Check sheet for the drawn part. Datum: minimum x, y, z corner. Units: mm. A direction names the side the tool comes from. Give positions to 0.01 mm unless a question says otherwise; leave off trailing zeros. Order: outer loops, then holes, each group sorted by start corner. A loop starts at its lowest first (then second) coordinate and runs counter-clockwise, first axis right, second up. Notation, with made-up numbers: (22.5, 81.5) -> (64.5, 81.5) arc R19 cw to (64.5, 92.5) -> close; hole circle Ø9 at (25.5, -33). An arc over 180 degrees is marked (long way). One line per question, with ' | ' between items. Start each with the question number.
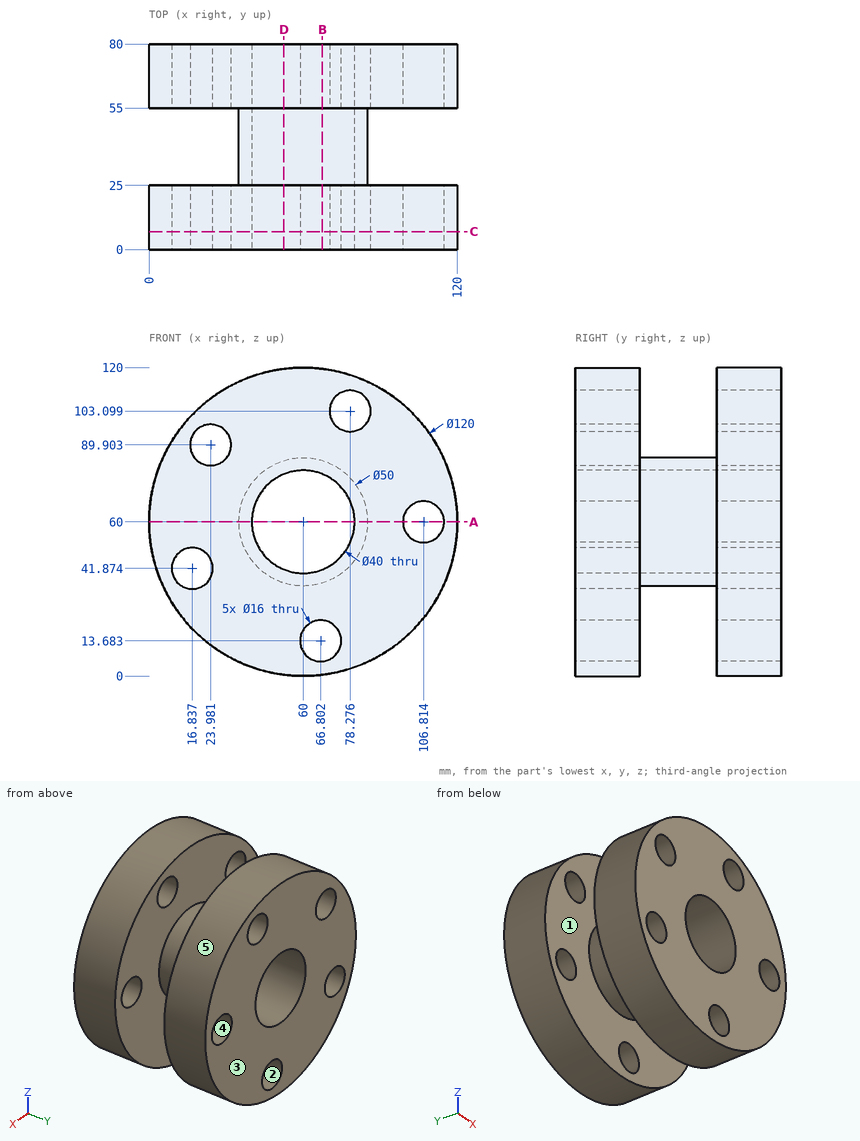
1. Cross-section at D-D on x = 52.5. Record the boundary of the cut face in (y, z).
2. Scan lines: probe 1 along Y at (x, z) = (79.5, 20); probe 2 along X at (y, z) = (68.5, 64.5) (1 decimal); probe 3 along Z at (x, y) = (20, 19.5) (1 decimal). Record each from-to range of solid material in increasing order.
3. Cross-section at C-C on y = 7. Record the boundary of the cut face in (x, z) (1 decimal), and give its area (3 significant figures).
4. Mould release check, pull along Z, two halves, no side actions. Record for the marked faces 3, 4 and 5: +Z half, -Z half, draft (parallel to the pull), parting line (faces both ways), or undercut.
5. Tool access check on the marked faces 1 and 2. Record the directions out of +Z, -Z, +X, -X, +Y, -Y that give a thin tool (end or side, any length) a straight path to the whole face; none if there is none.
6. Cross-section at B-B on x = 67.5. Record the boundary of the cut face in (y, z).
7. Cross-section at A-A on z = 60. Record the boundary of the cut face in (x, y) (1 decimal), and give its area (3 significant figures).
8. Go/stop test with flat-tipped pins: pin 1 (3 mm diameter, centred on x = 22.5, y = 25.5, fed in from +Z) (1 decimal); pin 2 (3 mm diameter, centred on y = 21, z = 103, fed in from -X); pin 3 (10 mm diameter, centred on x = 68, y = 14.5, fed in from -Z) (1 decimal). Record where each tip stops, or that it passes through.
Response values:
1) outline: (0, 0.47) -> (25, 0.47) -> (25, 36.15) -> (55, 36.15) -> (55, 0.47) -> (80, 0.47) -> (80, 41.46) -> (0, 41.46) -> close; (0, 78.54) -> (80, 78.54) -> (80, 119.53) -> (55, 119.53) -> (55, 83.85) -> (25, 83.85) -> (25, 119.53) -> (0, 119.53) -> close
2) probe 1: y = 0 to 25, 55 to 80 | probe 2: x = 0.2 to 40.5, 79.5 to 100.2, 113.4 to 119.8 | probe 3: z = 15.3 to 34.5, 49.2 to 83, 96.8 to 104.7
3) outline: circle Ø120 at (60, 60); hole circle Ø16 at (16.8, 41.9); hole circle Ø16 at (24, 89.9); hole circle Ø40 at (60, 60); hole circle Ø16 at (66.8, 13.7); hole circle Ø16 at (78.3, 103.1); hole circle Ø16 at (106.8, 60) | area: 9,050 mm²
4) face 3: draft | face 4: undercut | face 5: parting line
5) face 1: none | face 2: +Y, -Y
6) outline: (0, 0.47) -> (25, 0.47) -> (25, 5.71) -> (0, 5.71) -> close; (0, 21.65) -> (25, 21.65) -> (25, 36.15) -> (55, 36.15) -> (55, 21.65) -> (80, 21.65) -> (80, 41.46) -> (0, 41.46) -> close; (0, 78.54) -> (80, 78.54) -> (80, 119.53) -> (55, 119.53) -> (55, 83.85) -> (25, 83.85) -> (25, 119.53) -> (0, 119.53) -> close; (55, 0.47) -> (80, 0.47) -> (80, 5.71) -> (55, 5.71) -> close
7) outline: (0, 0) -> (40, 0) -> (40, 80) -> (0, 80) -> (0, 55) -> (35, 55) -> (35, 25) -> (0, 25) -> close; (80, 0) -> (98.8, 0) -> (98.8, 25) -> (85, 25) -> (85, 55) -> (98.8, 55) -> (98.8, 80) -> (80, 80) -> close; (114.8, 0) -> (120, 0) -> (120, 25) -> (114.8, 25) -> close; (114.8, 55) -> (120, 55) -> (120, 80) -> (114.8, 80) -> close | area: 3,500 mm²
8) pin 1: stops at z = 107.9 | pin 2: stops at x = 16.67 | pin 3: stops at z = 0.1
